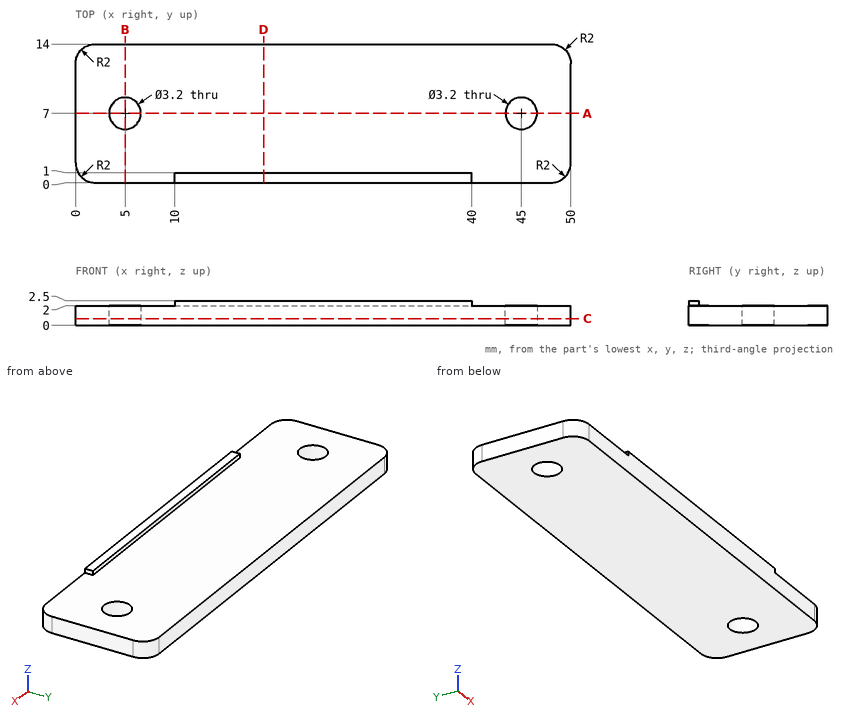
The figure shows three views and two pictorial views of one solid part (mm, origin at its lowest corner). Answer the questions. Coordinates: 2 decimals unless noted, no trailing zeros. Loops run counter-clockwise (first coordinate to the right, second up) from the corner with the lowest first, then second, coordinate; pieces in that order, holes last. Notation, with made-up numbers: M -29,42 L 23,42 A16 ccw 23,46 Z; hole C 16.25,-13 d7. An arc over 180 degrees is marked long. Use CSV: the item, a comma, the result in double quotes. Start each with the question number.
(1) Find section B-B, the plane x = 5. Give the vertices of the cut face in (y, z).
(2) Find section C-C, the plane z = 0.7. Give the vertices of the cut face in (x, y).
(3) Consider line 1 (Y direction, x = 45, z = 1.65); line 2 (Z direction, x = 25.5, y = 12.25); line 3 (X direction, y = 1.25, z = 1.4). Determine where each line is inside the solid, lowest interval first.
(4) Given pin 1 Ø4 at (x, y) = (45, 7) entering from +Z, flat-ended and moving along its own axis, determine where the tip first touches the part or whether it passes through.
(5) Find section D-D, the plane x = 19. Give the vertices of the cut face in (y, z).
(6) Find section A-A, the plane y = 7. Give the vertices of the cut face in (x, z).
Recorded:
1,outline,"M 0,0 L 5.4,0 L 5.4,2 L 0,2 Z; M 8.6,0 L 14,0 L 14,2 L 8.6,2 Z"
2,outline,"M 0,2 A2 ccw 2,0 L 48,0 A2 ccw 50,2 L 50,12 A2 ccw 48,14 L 2,14 A2 ccw 0,12 Z; hole C 5,7 d3.2; hole C 45,7 d3.2"
3,line 1,"y = 0 to 5.4, 8.6 to 14"
3,line 2,"z = 0 to 2"
3,line 3,"x = 0.15 to 49.85"
4,pin 1,"stops at z = 2"
5,outline,"M 0,0 L 14,0 L 14,2 L 1,2 L 1,2.5 L 0,2.5 Z"
6,outline,"M 0,0 L 3.4,0 L 3.4,2 L 0,2 Z; M 6.6,0 L 43.4,0 L 43.4,2 L 6.6,2 Z; M 46.6,0 L 50,0 L 50,2 L 46.6,2 Z"
